Input: dimensioned drawing with shaded views. Units: mm. Origin: part minimum x, y, z. A direction names the side the tool comes from. Give positions to 0.01 mm unless a question says otherwise; leave off trailing zeros. Write each loop counter-clockwise with the first axis right and the second up, starting at its lowest first coordinate (ties: lowest second). Pieces come first, ordered by that corner, then holes.
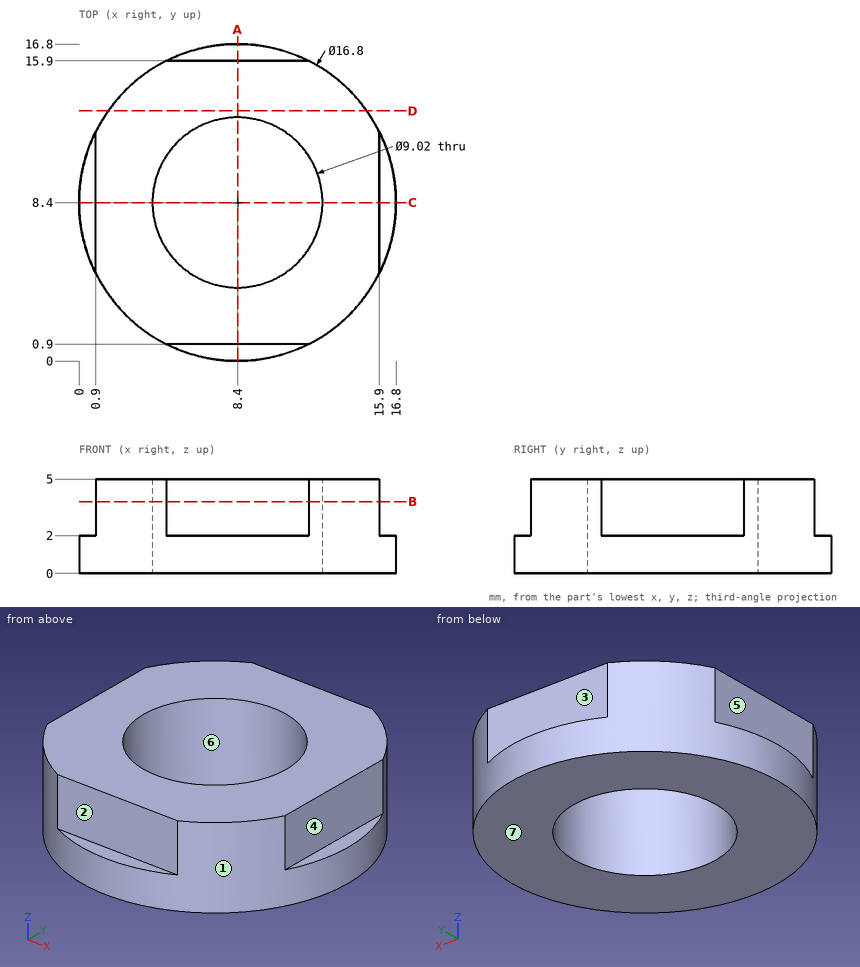
Item 1: Section A-A, the plane x = 8.4. Return the cut outline in (y, z).
Found:
outline: (0, 0) - (3.89, 0) - (3.89, 5) - (0.9, 5) - (0.9, 2) - (0, 2) - close; (12.91, 0) - (16.8, 0) - (16.8, 2) - (15.9, 2) - (15.9, 5) - (12.91, 5) - close
Item 2: Section B-B, the plane z = 3.8. Return the cut outline in (x, y).
Found:
outline: (0.9, 4.62) arc R8.4 ccw to (4.62, 0.9) - (12.18, 0.9) arc R8.4 ccw to (15.9, 4.62) - (15.9, 12.18) arc R8.4 ccw to (12.18, 15.9) - (4.62, 15.9) arc R8.4 ccw to (0.9, 12.18) - close; hole circle Ø9.02 at (8.4, 8.4)
Item 3: Pin query (flat end, axial travel): pin 1 Ø1.5 at (y, z) = (8, 4) entering from -X; pin 2 Ø1.5 at (y, z) = (7.5, 3.5) entering from +X; pin 3 Ø0.5 at (x, y) = (8.5, 0) entering from +Z; pin 4 Ø8 at (x, y) = (8.4, 8.4) entering from -Z. Return the tip coordinate at first contact, or that it passes through.
Found:
pin 1: stops at x = 0.9
pin 2: stops at x = 15.9
pin 3: stops at z = 2
pin 4: passes through
Item 4: Reachability of the marked faces 1, 2 and 3 from +Z, -Z, +X, -X, +Y, -Y: full face, straight path, thin tool, end or side. Return the list, or none.
Found:
face 1: +Z, -Z
face 2: +Z, +X, -X, -Y
face 3: +Z, +X, -X, +Y
Item 5: Pull-direction query (X, two-part tool) for the marked faces 4, 5, 6 and 7; classes: +X half, -X half, draft (parallel to the pull), parting line (faces both ways), or undercut.
Found:
face 4: +X half
face 5: -X half
face 6: undercut
face 7: draft
Item 6: Section D-D, the plane y = 13.25. Return the cut outline in (x, z), plus the area to 3 significant figures.
Found:
outline: (1.54, 0) - (15.26, 0) - (15.26, 5) - (1.54, 5) - close
area: 68.6 mm2
Item 7: Line query: L1, parallel to Y at x = 8.4, z = 3.7; L2, parallel to Y at x = 8.4, z = 1.6; L3, parallel to X at y = 10, z = 1.45. Output: solid intervals per line, ascending.
Found:
L1: y = 0.9 to 3.89, 12.91 to 15.9
L2: y = 0 to 3.89, 12.91 to 16.8
L3: x = 0.15 to 4.18, 12.62 to 16.65
